from build123d import *

# Parameters (mm, degrees)
F1_DEPTH      = 12.5
F1_DEPTH_BACK = 12.5
F3_DEPTH      = 190
F3_DEPTH_BACK = 190
F5_DEPTH      = 75
F7_DEPTH      = 75
F8_R          = 11
F9_DEPTH      = 25


with BuildPart() as f1:
    # F0 (on Top) → F1 (new body, two sides)
    with BuildSketch(Plane.XY) as f1_sk:
        Polygon((105, 101), (-105, 101), (-190, -44), (-190, -101), (-115, -101), (-115, -76), (115, -76), (115, -101), (190, -101), (190, -44), align=None)
    extrude(amount=F1_DEPTH)
    extrude(f1_sk.sketch, amount=-F1_DEPTH_BACK)

    # F2 (on Right) → F3 (cut, two sides)
    with BuildSketch(Plane.YZ) as f3_sk:
        Polygon((-92, 12.5), (-101, 12.5), (-101.165957, -12.499449), align=None)
    extrude(amount=F3_DEPTH, mode=Mode.SUBTRACT)
    extrude(f3_sk.sketch, amount=-F3_DEPTH_BACK, mode=Mode.SUBTRACT)

    # F4 (on face) → F5 (cut, through all)
    with BuildSketch(Plane.YZ.offset(-115)):
        Polygon((-72.852649, -0.5), (-96.766403, -0.5), (-101.166159, -12.5), (-71.166159, -12.5), align=None)
    extrude(amount=-F5_DEPTH, mode=Mode.SUBTRACT)

    # F6 (on face) → F7 (cut, through all)
    with BuildSketch(Plane(origin=(115, 0, 0), x_dir=(0, -1, 0), z_dir=(-1, 0, 0))):
        Polygon((101.166159, -12.5), (96.766403, -0.5), (72.92292, 0), (71.166159, -12.5), align=None)
    extrude(amount=-F7_DEPTH, mode=Mode.SUBTRACT)

    # F8 (on face) → F9 (cut)
    with BuildSketch(Plane(origin=(0, 0, -12.5), x_dir=(1, 0, 0), z_dir=(0, 0, -1))):
        with Locations((-80, -73)):
            Circle(F8_R)
        with Locations((-80, 2)):
            Circle(F8_R)
        with Locations((80, -73)):
            Circle(F8_R)
        with Locations((80, 2)):
            Circle(F8_R)
    extrude(amount=-F9_DEPTH, mode=Mode.SUBTRACT)


solid = f1.part
Design review of the part built by this model. Coordinates are the model's own, in mm. A direction names the side the tool comes from. Round coordinates to 2 decimals unless told otherwise and drop trailing zeros. Write each loop counter-clockwise with the first axis right and the second up, starting at its lowest first coordinate (ties: lowest second). Pieces come first, ordered by that corner, then holes.
Item 1: Draft analysis for pull direction X (two halves, no side actions). For faces 4 (the flat face through (190, -65, 3)), 5 (the flat face through (1, 101, 0)), 6 (the flat face through (-2, -76, 0)), state which applies: released by +X, released by -X, zero draft, split by the parting line, or undercut.
Item 2: Wall thickness on L1, parallel to Y at x = 80, z = -1.75; L2, parallel to X at y = 73, z = -5; L3, parallel to X at y = -2, z = -2: over which ranges is each line inside the solid? List them lowest first.
Item 3: For faces 1 (the cylindrical face through (69, 73, 0)), 2 (the flat face through (-115, -84, 6)), 3 (the flat face through (-151.98, -72, -6.58)), list the 3-axis set-ups (+Z, -Z, +X, -X, +Y, -Y) from which the entire face can be reached by the end or side of a thin tool; tool diameter is ignored.
Item 4: For pin 1 Ø1.5 at (y, z) = (-74, -9) entering from +X; pin 2 Ø10 at (y, z) = (20, -9.5) entering from -X; pin 3 Ø8 at (y, z) = (-24, 9) entering from -X, all flat-tipped, find the tip position at first contact; note any pin that passes through.
Item 5: Consider section D-D on z = -8.5. Give the boundary of the cut face in (x, y).
Item 6: Consider section A-A on x = -80. Give the boundary of the cut face in (y, z).
Item 7: Consider section B-B on y = -80. Give the boundary of the cut face in (x, z).
Item 8: Consider section C-C on y = 73. Give the boundary of the cut face in (x, z), and give its area (3 significant figures).
Check values:
1. face 4: released by +X
1. face 5: zero draft
1. face 6: undercut
2. L1: y = -76 to -13, 9 to 62, 84 to 101
2. L2: x = -121.41 to -91, -69 to 69, 91 to 121.41
2. L3: x = -165.38 to -91, -69 to 69, 91 to 165.38
3. face 1: +Z, -Z
3. face 2: +Z, -Z, -Y
3. face 3: -Z, -X, -Y
4. pin 1: stops at x = 115
4. pin 2: stops at x = -155.41
4. pin 3: stops at x = -180.62
5. outline: (-190, -71.73) - (-115, -71.73) - (-115, -76) - (115, -76) - (115, -71.73) - (190, -71.73) - (190, -44) - (105, 101) - (-105, 101) - (-190, -44) - close; hole circle Ø22 at (-80, -2); hole circle Ø22 at (-80, 73); hole circle Ø22 at (80, -2); hole circle Ø22 at (80, 73)
6. outline: (-76, -12.5) - (-13, -12.5) - (-13, 12.5) - (-76, 12.5) - close; (9, -12.5) - (62, -12.5) - (62, 12.5) - (9, 12.5) - close; (84, -12.5) - (101, -12.5) - (101, 12.5) - (84, 12.5) - close
7. outline: (-190, -0.5) - (-115, -0.5) - (-115, 12.5) - (-190, 12.5) - close; (115, -0.15) - (190, -0.15) - (190, 12.5) - (115, 12.5) - close
8. outline: (-121.41, -12.5) - (-91, -12.5) - (-91, 12.5) - (-121.41, 12.5) - close; (-69, -12.5) - (69, -12.5) - (69, 12.5) - (-69, 12.5) - close; (91, -12.5) - (121.41, -12.5) - (121.41, 12.5) - (91, 12.5) - close
8. area: 4,970 mm2
